Geometry: see drawing. Coordinates: mm, zero at the bounding-box minimum. Coordinates: 2 decimals unless noted, no trailing zeros. Write each loop counter-clockwise with the first axis right and the second up, starting at its lowest first coordinate (ties: lowest second). Pieces come first, ordered by that corner, then holes. Notation, with made-up numbers: M 83,-1 L 107,-1 A28 cw 107,36 Z; hole C 31.5,46.25 d1. An arc over 180 degrees is marked long. Write item = value, one per line. Start each with the question number.
1. Section query B-B (y = 22.5). Output: boundary loops of the cut face in (x, z).
2. Line query: line 1 along X through (y, z) = (228.5, 1.5) (1 decimal); line 2 along Y through (x, z) = (52, 5.5) (1 decimal); line 3 along X through (y, z) = (54, 0.5) (1 decimal). Output: solid intervals per line, ascending.
3. Pin query (flat end, axial travel): pin 1 Ø13.5 at (x, y) = (57.65, 227.35) entering from -Z. Return the tip coordinate at first contact, or that it passes through.
4. Section query C-C (z = 4). Give the number of separate pieces and of enclosed holes in the cut face, then the cut area to 3 significant figures.
5. Section query A-A (x = 142.5). Output: boundary loops of the cut face in (y, z).
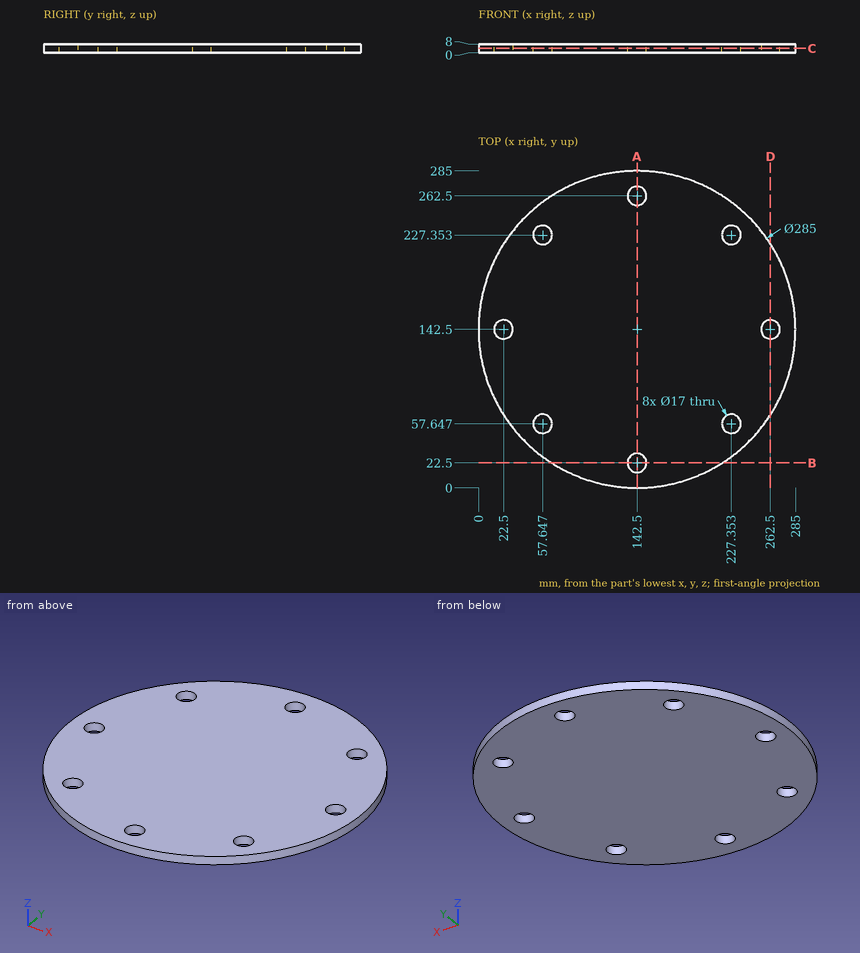
Results are:
q1.outline = M 65.65,0 L 134,0 L 134,8 L 65.65,8 Z; M 151,0 L 219.35,0 L 219.35,8 L 151,8 Z
q2.line_1 = 28.9 to 49.2, 66.1 to 218.9, 235.8 to 256.1
q2.line_2 = 32.4 to 51.3, 64 to 221, 233.7 to 252.6
q2.line_3 = 30.8 to 50, 65.3 to 219.7, 235 to 254.2
q3.pin_1 = through
q4.separate_pieces = 1
q4.enclosed_holes = 8
q4.area = 62,000 mm^2
q5.outline = M 0,0 L 14,0 L 14,8 L 0,8 Z; M 31,0 L 254,0 L 254,8 L 31,8 Z; M 271,0 L 285,0 L 285,8 L 271,8 Z
